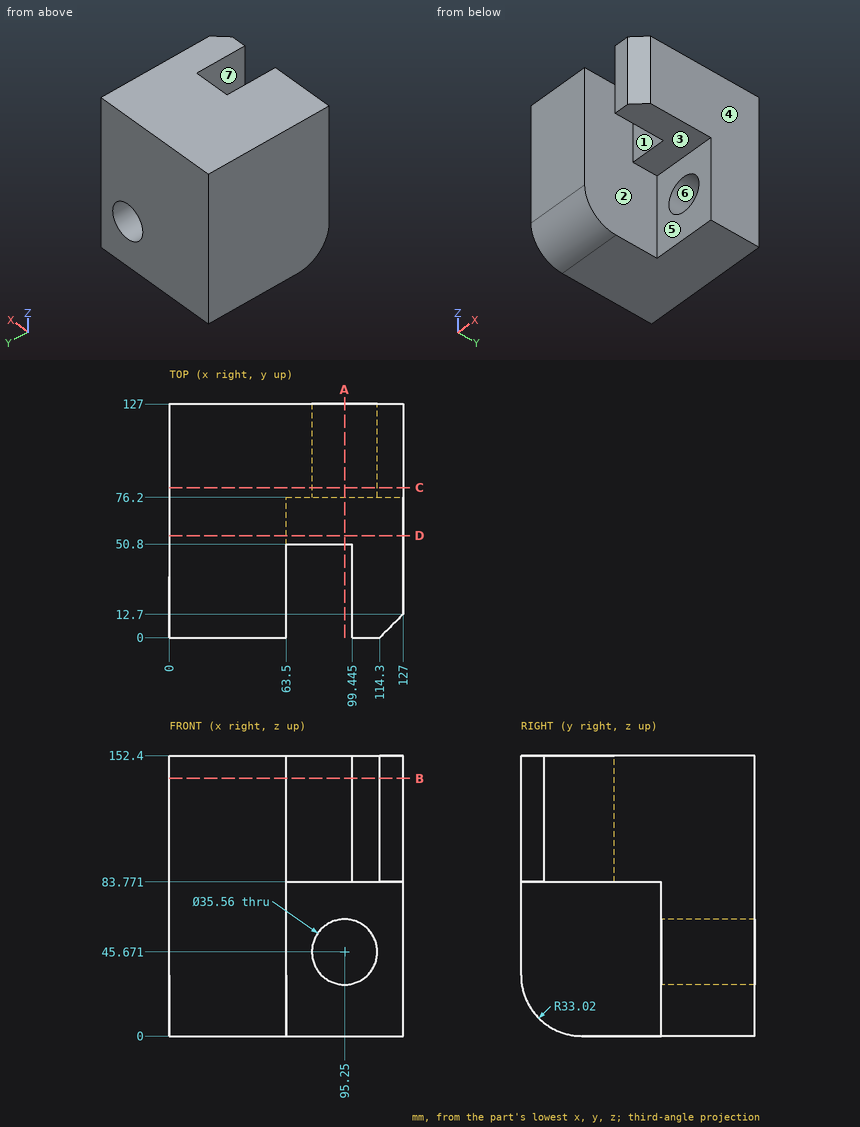
Here's the drawing with two shaded views (mm, measured from the low corner). I have some questions. A direction names the side the tool comes from. Coordinates: 2 decimals unless noted, no trailing zeros. Loops run counter-clockwise (first coordinate to the right, second up) from the corner with the lowest first, then second, coordinate; pieces in that order, holes last. Notation, with made-up numbers: M 61,2 L 116,2 A22 ccw 116,10 Z; hole C 58,39.5 d2. An arc over 180 degrees is marked long. Put each result on its own line as item: value. Start each with the question number.
(1) Will these pins go through, and if not, where does the flat tip stop? pin 1 Ø18 at (x, z) = (77.5, 111.5) entering from -Y; pin 2 Ø15 at (y, z) = (28, 102) entering from -X; pin 3 Ø4 at (x, z) = (106.5, 21.5) entering from -Y; pin 4 Ø19 at (x, y) = (101, 21.5) entering from -Z.
(2) Imagine slicing it at A-A on x = 95.25. List the corners of the cut face in (y, z) for me.
(3) I need wall thicknesses on probe 1 along Z at (x, y) = (95, 87); probe 2 along Z at (x, y) = (117.5, 5); probe 3 along X at (y, z) = (121.5, 49) (1 decimal). Which ranges of each line are inside material? Lowest first, please.
(4) We'd pull the mould along X, two halves only. Please class the marked faces 4, 5, 6 and 7: +X half, -X half, draft (parallel to the pull), parting line (faces both ways), or undercut.
(5) Which directions (+Z, -Z, +X, -X, +Y, -Y) give clear straight access to the entire face, cutting with the end or side of a thin tool? Please do the marked faces 1, 2 and 3.
(6) Imagine slicing it at C-C on y = 81.5. List the corners of the cut face in (x, z) for me.
(7) Imagine slicing it at B-B on z = 140. List the corners of the cut face in (x, y) for me (1 decimal).
(8) Imagine slicing it at D-D on y = 55.5. List the corners of the cut face in (x, z) for me.
Worked answers:
1. pin 1: stops at y = 50.8
1. pin 2: stops at x = 0
1. pin 3: stops at y = 76.2
1. pin 4: stops at z = 83.77
2. outline: M 50.8,83.77 L 76.2,83.77 L 76.2,63.45 L 127,63.45 L 127,152.4 L 50.8,152.4 Z; M 76.2,0 L 127,0 L 127,27.89 L 76.2,27.89 Z
3. probe 1: z = 0 to 27.89, 63.45 to 152.4
3. probe 2: z = 83.77 to 152.4
3. probe 3: x = 0 to 77.8, 112.7 to 127
4. face 4: +X half
4. face 5: draft
4. face 6: undercut
4. face 7: undercut
5. face 1: +Z, -Z, -Y
5. face 2: -Z, -Y
5. face 3: -Z, +X, -Y
6. outline: M 0,0 L 127,0 L 127,152.4 L 0,152.4 Z; hole C 95.25,45.67 d35.56
7. outline: M 0,0 L 63.5,0 L 63.5,50.8 L 99.4,50.8 L 99.4,0 L 114.3,0 L 127,12.7 L 127,127 L 0,127 Z
8. outline: M 0,0 L 63.5,0 L 63.5,83.77 L 127,83.77 L 127,152.4 L 0,152.4 Z
